```python
from build123d import *

# Parameters (mm, degrees)
SKETCH1_R           = 14.2875
SKETCH1_R_2         = 3.2639
SKETCH1_R_3         = 2.4892
SKETCH1_R_4         = 12.7
BOSS_EXTRUDE1_DEPTH = 6.35
FILLET1_R           = 12.7
CUT_EXTRUDE1_DEPTH  = 1118.158262331
FILLET2_R           = 3.175


with BuildPart() as part:
    # Sketch1 → Boss-Extrude1 (new body)
    with BuildSketch(Plane(origin=(0, 0, 0), x_dir=(0, 0, -1), z_dir=(1, 0, 0))):
        with BuildLine():
            ThreePointArc((-977.470329324, 488.018353149), (-979.865093402, 482.854765121), (-977.16025221, 477.846634687))
            Line((-977.16025221, 477.846634687), (-964.636474603, 469.0773912))
            ThreePointArc((-964.636474603, 469.0773912), (-960.124717731, 449.073600219), (-940.590272736, 442.835566684))
            Line((-940.590272736, 442.835566684), (-904.317406585, 380.009119575))
            ThreePointArc((-904.317406585, 380.009119575), (-899.31875, 348.305993858), (-869.363709458, 359.828593129))
            Line((-869.363709458, 359.828593129), (-793.75, 359.828593129))
            ThreePointArc((-793.75, 359.828593129), (-788.33277515, 362.865562051), (-788.097264793, 369.071530162))
            Line((-788.097264793, 369.071530162), (-828.71050777, 448.428911911))
            ThreePointArc((-828.71050777, 448.428911911), (-824.098459608, 455.475832937), (-822.685744308, 463.778502368))
            Line((-822.685744308, 463.778502368), (-790.971974231, 475.344799559))
            ThreePointArc((-790.971974231, 475.344799559), (-754.671988994, 483.059997875), (-783.134686327, 506.873608979))
            Line((-783.134686327, 506.873608979), (-807.984116899, 534.429271156))
            ThreePointArc((-807.984116899, 534.429271156), (-810.119275968, 535.978683887), (-812.699834325, 536.526682631))
            Line((-812.699834325, 536.526682631), (-848.620858809, 536.526682631))
            ThreePointArc((-848.620858809, 536.526682631), (-850.667304495, 536.18788551), (-852.495378558, 535.207646428))
            Line((-852.495378558, 535.207646428), (-873.874828732, 518.742590175))
            ThreePointArc((-873.874828732, 518.742590175), (-875.286935498, 517.920433239), (-876.862092968, 517.485845513))
            Line((-876.862092968, 517.485845513), (-952.412407774, 506.824976977))
            ThreePointArc((-952.412407774, 506.824976977), (-954.033002966, 506.371065297), (-955.477439746, 505.507371499))
            Line((-955.477439746, 505.507371499), (-977.470329324, 488.018353149))
        make_face()
        with Locations((-774.7, 488.038469669)):
            Circle(SKETCH1_R, mode=Mode.SUBTRACT)
        with Locations((-843.309156693, 463.016093129)):
            Circle(SKETCH1_R, mode=Mode.SUBTRACT)
        with Locations((-889, 366.178593129)):
            Circle(SKETCH1_R, mode=Mode.SUBTRACT)
        with Locations((-944.909156693, 463.016093129)):
            Circle(SKETCH1_R, mode=Mode.SUBTRACT)
        with Locations((-850.9, 366.178593129)):
            Circle(SKETCH1_R_2, mode=Mode.SUBTRACT)
        with Locations((-831.85, 366.178593129)):
            Circle(SKETCH1_R_2, mode=Mode.SUBTRACT)
        with Locations((-812.8, 366.178593129)):
            Circle(SKETCH1_R_2, mode=Mode.SUBTRACT)
        with Locations((-793.75, 366.178593129)):
            Circle(SKETCH1_R_2, mode=Mode.SUBTRACT)
        with Locations((-973.518041839, 483.048250169)):
            Circle(SKETCH1_R_2, mode=Mode.SUBTRACT)
        with Locations((-951.525152262, 500.537268519)):
            Circle(SKETCH1_R_2, mode=Mode.SUBTRACT)
        with Locations((-868.760346567, 512.216170389)):
            Circle(SKETCH1_R_2, mode=Mode.SUBTRACT)
        with Locations((-848.620858809, 494.255658147)):
            Circle(SKETCH1_R_3, mode=Mode.SUBTRACT)
        with Locations((-812.699834325, 494.255658147)):
            Circle(SKETCH1_R_3, mode=Mode.SUBTRACT)
        with Locations((-830.660346567, 512.216170389)):
            Circle(SKETCH1_R_4, mode=Mode.SUBTRACT)
        with Locations((-848.620858809, 530.176682631)):
            Circle(SKETCH1_R_3, mode=Mode.SUBTRACT)
        with Locations((-812.699834325, 530.176682631)):
            Circle(SKETCH1_R_3, mode=Mode.SUBTRACT)
    extrude(amount=BOSS_EXTRUDE1_DEPTH)

    # Fillet1
    fillet1_edges = [part.edges().sort_by_distance(p)[0] for p in [
        (3.175, 475.344799559, 790.971974231),
        (3.175, 463.778502368, 822.685744308),
        (3.175, 448.428911911, 828.71050777),
        (3.175, 359.828593129, 869.363709458),
        (3.175, 380.009119575, 904.317406585),
        (3.175, 442.835566684, 940.590272736),
        (3.175, 469.0773912, 964.636474603),
    ]]
    fillet(fillet1_edges, radius=FILLET1_R)

    # Sketch2 → Cut-Extrude1 (cut, through all)
    with BuildSketch(Plane(origin=(6.35, 0, 0), x_dir=(0, 0, -1), z_dir=(1, 0, 0))):
        with BuildLine():
            Line((-948.926016287, 494.491122688), (-962.909028761, 483.371657877))
            Line((-962.909028761, 483.371657877), (-957.352053862, 479.480622163))
            ThreePointArc((-957.352053862, 479.480622163), (-944.524975807, 483.650016927), (-931.861993278, 479.00602537))
            Line((-931.861993278, 479.00602537), (-896.429960387, 501.898815853))
            Line((-896.429960387, 501.898815853), (-948.926016287, 494.491122688))
        make_face()
        with BuildLine():
            Line((-857.971369961, 477.539381611), (-871.187574345, 503.08782473))
            Line((-871.187574345, 503.08782473), (-914.338399947, 475.207888722))
            ThreePointArc((-914.338399947, 475.207888722), (-915.66067146, 471.642886863), (-912.615371721, 469.366093129))
            Line((-912.615371721, 469.366093129), (-862.945447235, 469.366093129))
            ThreePointArc((-862.945447235, 469.366093129), (-860.938606544, 473.744974907), (-857.971369961, 477.539381611))
        make_face()
        with BuildLine():
            ThreePointArc((-925.272866151, 456.666093129), (-927.036557422, 452.697343129), (-929.591750108, 449.185566684))
            Line((-929.591750108, 449.185566684), (-893.318883957, 386.359119575))
            ThreePointArc((-893.318883957, 386.359119575), (-889.853529885, 386.798435344), (-886.363723266, 386.647018844))
            Line((-886.363723266, 386.647018844), (-857.431129838, 447.966964226))
            ThreePointArc((-857.431129838, 447.966964226), (-860.739698931, 451.966993458), (-862.945447235, 456.666093129))
            Line((-862.945447235, 456.666093129), (-925.272866151, 456.666093129))
        make_face()
        with BuildLine():
            Line((-804.13305316, 372.528593129), (-840.015978185, 442.643037846))
            ThreePointArc((-840.015978185, 442.643037846), (-842.977262335, 442.381262081), (-845.945433426, 442.547667414))
            Line((-845.945433426, 442.547667414), (-874.878026855, 381.227722032))
            ThreePointArc((-874.878026855, 381.227722032), (-871.569457762, 377.2276928), (-869.363709458, 372.528593129))
            Line((-869.363709458, 372.528593129), (-804.13305316, 372.528593129))
        make_face()
    extrude(amount=-CUT_EXTRUDE1_DEPTH, mode=Mode.SUBTRACT)

    # Fillet2
    fillet2_edges = [part.edges().sort_by_distance(p)[0] for p in [
        (3.175, 479.00602537, 931.861993278),
        (3.175, 479.480622163, 957.352053862),
        (3.175, 483.371657877, 962.909028761),
        (3.175, 494.491122688, 948.926016287),
        (3.175, 501.898815853, 896.429960387),
        (3.175, 386.647018844, 886.363723266),
        (3.175, 386.359119575, 893.318883957),
        (3.175, 449.185566684, 929.591750108),
        (3.175, 456.666093129, 925.272866151),
        (3.175, 456.666093129, 862.945447235),
        (3.175, 447.966964226, 857.431129838),
        (3.175, 372.528593129, 869.363709458),
        (3.175, 381.227722032, 874.878026855),
        (3.175, 442.547667414, 845.945433426),
        (3.175, 442.643037846, 840.015978185),
        (3.175, 372.528593129, 804.13305316),
        (3.175, 503.08782473, 871.187574345),
        (3.175, 477.539381611, 857.971369961),
        (3.175, 469.366093129, 862.945447235),
        (3.175, 506.873608979, 783.134686327),
    ]]
    fillet(fillet2_edges, radius=FILLET2_R)


solid = part.part
```
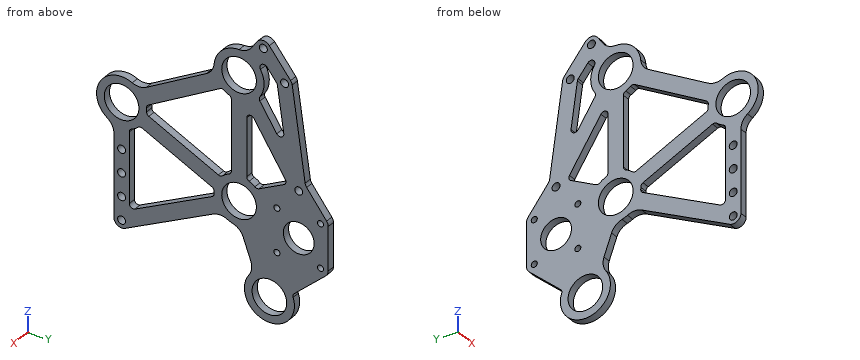
Build history of the part. All positions in model axes, mm. Coordinates: 2 decimals unless noted, no trailing zeros. Order: outer loops, then holes, each group sorted by start corner. A loop starts at its lowest first (then second) coordinate and runs counter-clockwise, first axis right, second up.
Item 1: Drill centre lines: L1, parallel to Y at x = 2.25, z = 774.7; L2, parallel to Z at x = 6.25, y = 409; L3, parallel to Y at x = 3.25, z = 889. Where is each one in solid material? Low to high.
Filled in:
L1: y = 467.4 to 473.75, 502.33 to 508.68
L2: z = 808.53 to 822.8, 861.77 to 875.82, 906.39 to 921.06
L3: y = 345.54 to 351.89, 380.47 to 386.82, 456.67 to 469.37, 491.58 to 515.77
Item 2: Drop flat-ended pins along their axis: pin 1 Ø3 at (x, z) = (3, 877.5) entering from +Y; pin 2 Ø3 at (x, y) = (3.5, 373) entering from +Z. Give the stop position or say it passes through.
Filled in:
pin 1: stops at y = 517.67
pin 2: stops at z = 908.94
Item 3: Saw through at B-B on y = 396.5. List the corners of the cut face in (x, z), then the cut area to 3 significant figures.
Filled in:
outline: (0, 802.13) - (6.35, 802.13) - (6.35, 816.4) - (0, 816.4) - close; (0, 867.67) - (6.35, 867.67) - (6.35, 881.71) - (0, 881.71) - close; (0, 899.17) - (6.35, 899.17) - (6.35, 913.84) - (0, 913.84) - close
area: 273 mm2
Item 4: Saw through at D-D on x = 2. State how many separate pieces and enclosed holes the cut face has, then the cut area to 3 significant figures.
Filled in:
separate pieces: 1
enclosed holes: 20
area: 13,300 mm2
Item 5: Saw through at C-C on z = 831.85. List the corners of the cut face in (x, y), then the cut area to 3 significant figures.
Filled in:
outline: (0, 359.83) - (6.35, 359.83) - (6.35, 362.91) - (0, 362.91) - close; (0, 369.44) - (6.35, 369.44) - (6.35, 372.53) - (0, 372.53) - close; (0, 426.69) - (6.35, 426.69) - (6.35, 454.48) - (0, 454.48) - close; (0, 471.55) - (6.35, 471.55) - (6.35, 499.57) - (0, 499.57) - close; (0, 524.86) - (6.35, 524.86) - (6.35, 536.53) - (0, 536.53) - close
area: 468 mm2
Item 6: Saw through at A-A on z = 774.7. List the corners of the cut face in (x, y).
Filled in:
outline: (0, 467.4) - (6.35, 467.4) - (6.35, 473.75) - (0, 473.75) - close; (0, 502.33) - (6.35, 502.33) - (6.35, 508.68) - (0, 508.68) - close
